Can you work these out from the model? Positions are in its coordinate system, mm. Give positions to 0.01 mm unless a question says otherwise; leave off trailing zeros. Write each loop counter-clockwise with the first axis right and the second up, starting at its lowest first coordinate (ties: lowest second). Pieces come first, ordered by that corner, then holes.
from build123d import *

# Parameters (mm, degrees)
SKETCH1_R               = 6.35
BOSS_EXTRUDE1_DEPTH     = 83.82
SKETCH3_R               = 4.445
BOSS_EXTRUDE2_DEPTH     = 25.4
FILLET1_R               = 3.81
CUT_EXTRUDE1_DEPTH      = 7.62
CUT_EXTRUDE1_DEPTH_BACK = 7.62
SKETCH4_R               = 3.2385
FILLET2_R               = 0.508


with BuildPart() as part:
    # Sketch1 → Boss-Extrude1 (new body)
    with BuildSketch(Plane(origin=(0, 0, 0), x_dir=(1, 0, 0), z_dir=(0, 1, 0))):
        with Locations(Location((0, 0, 0), (0, 0, 270))):
            Circle(SKETCH1_R)
    extrude(amount=BOSS_EXTRUDE1_DEPTH)

    # Sketch3 → Boss-Extrude2 (add)
    with BuildSketch(Plane(origin=(0, 0, 0), x_dir=(1, 0, 0), z_dir=(0, 1, 0))):
        with Locations(Location((0, 0, 0), (0, 0, 270))):
            Circle(SKETCH3_R)
    extrude(amount=-BOSS_EXTRUDE2_DEPTH)

    # Fillet1
    # the kernel refuses this fillet: 3.81 mm, written as the material it adds along each edge
    with BuildSketch(Plane(origin=(0, 0, 0), x_dir=(0, 0, 1), z_dir=(-1, 0, 0))) as fillet1_piece_1:
        with BuildLine():
            CenterArc((8.255, -3.299556788), FILLET1_R, 120, 60)
            Line((4.445, -3.299556788), (4.3688, -3.299556788))
            Line((4.3688, -3.299556788), (4.3688, 0))
            Line((4.3688, 0), (4.445, 0.0762))
            ThreePointArc((4.445, 0.0762), (5.3975, 0.0762), (6.3119, 0.065991136))
            Line((6.3119, 0.065991136), (6.35, 0))
        make_face()
    revolve(axis=Axis((0, 0, 0), (0, 1, 0)))

    # Sketch4 → Cut-Extrude1 (cut, two sides: drawn at the far end of the back side and taken through both)
    with BuildSketch(Plane(origin=(0, 0, 0), x_dir=(0, 0, -1), z_dir=(1, 0, 0)).offset(-CUT_EXTRUDE1_DEPTH_BACK)):
        with Locations((0, -25.4)):
            Circle(SKETCH4_R)
    extrude(amount=CUT_EXTRUDE1_DEPTH + CUT_EXTRUDE1_DEPTH_BACK, mode=Mode.SUBTRACT)

    # Fillet2
    fillet2_edges = [part.edges().sort_by_distance(p)[0] for p in [
        (0, -25.4, -3.2385),
        (0, -25.4, 3.2385),
        (0, 0, -6.35),
    ]]
    fillet(fillet2_edges, radius=FILLET2_R)


solid = part.part
(1) Will these pins go through, and if not, where does the flat tip stop? P1, Ø1, axis at x = -4, y = 65, coming from the -Z side; P2, Ø1, axis at y = 8, z = -5, coming from the +X side; P3, Ø1, axis at y = 59.5, z = -2.5, coming from the +X side.
Returned:
P1: stops at z = -5.3
P2: stops at x = 4.48
P3: stops at x = 6.03
(2) If I drill on L1, parallel to X at y = 23, z = -0.25; L2, parallel to Y at x = -3.5, z = -5; L3, parallel to Z at x = -4, y = 54.5, over which ranges is the centre line in solid material (lowest first)?
Returned:
L1: x = -6.35 to 6.35
L2: y = -0.16 to 83.82
L3: z = -4.93 to 4.93
(3) Imagine slicing it at A-A, the plane y = -13.5. Write out the boundary of the cut face in (x, z) (3 decimals).
Returned:
outline: circle Ø8.89 at (0, 0)
(4) If we mould it in two halves opening along Z, with no side actions, what happens to faces 1 (the face through (-0.062, -22.162, -0.065)), 2 (the face through (-2.432, 41.466, 5.866)), 3 (the face through (0, 83.82, 0))? For each: +Z half, -Z half, draft (parallel to the pull), parting line (faces both ways), or undercut.
Returned:
face 1: undercut
face 2: parting line
face 3: draft
(5) Imagine slicing it at B-B, the plane y = 55. Write out the boundary of the cut face in (x, z), plus the area to 3 significant figures.
Returned:
outline: circle Ø12.7 at (0, 0)
area: 127 mm2
